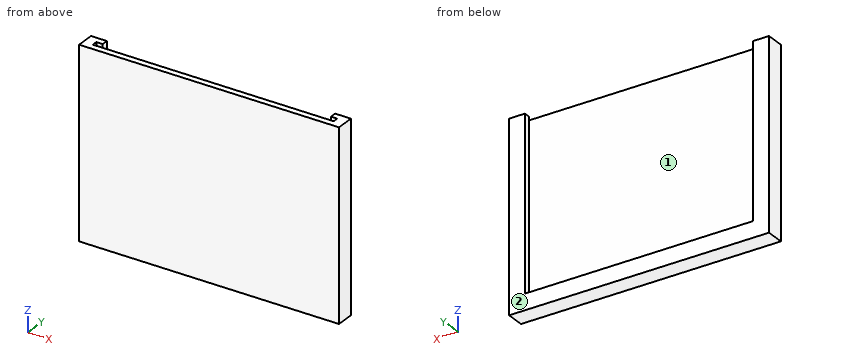
Autodesk Inventor part; units mm, degrees
ref_plane "YZ Plane" through (0, 0, 0) normal (1, 0, 0) x (0, 1, 0)
ref_plane "XZ Plane" through (0, 0, 0) normal (0, 1, 0) x (-1, 0, 0)
ref_plane "XY Plane" through (0, 0, 0) normal (0, 0, 1) x (1, 0, 0)
sketch "Szkic1" plane through (0, 0, 0) normal (0, 1, 0) x (-1, 0, 0)
  line L0 (7, 46.073) -> (-75, 46.073)
  line L1 (-75, 46.073) -> (-75, -13)
  line L2 (-75, -13) -> (7, -13)
  line L3 (7, -13) -> (7, 46.073)
  point P0 (0, 0)
  dimension "d0" = 82
  dimension "d1" = 59.073
extrude "Wyciągnięcie proste1" add sketch "Szkic1" along normal blind 2
sketch "Szkic2" plane through (0, 2, 0) normal (0, 1, 0) x (1, 0, 0)
  line L0 (75, -46.073) -> (75, 13)
  line L1 (75, 13) -> (-7, 13)
  line L2 (-7, 13) -> (-7, -46.073)
  line L3 (-7, -46.073) -> (75, -46.073)
  line L4 (-4, 10) -> (72, 10)
  line L5 (72, 10) -> (72, -43.073)
  line L6 (72, -43.073) -> (-4, -43.073)
  line L7 (-4, -43.073) -> (-4, 10)
  line L8 (-4, -43.073) -> (-4, -46.073)
  line L9 (72, -43.073) -> (72, -46.073)
  line L10 (-7, -46.073) -> (75, -46.073)
  point P0 (0, 0)
  dimension "d4" = 3
extrude "Wyciągnięcie proste2" add sketch "Szkic2" along normal blind 1.7 contours L3 L9 L5 L4 L7 L8 L2 L1 L0
sketch "Szkic3" plane through (0, 3.7, 0) normal (0, 1, 0) x (1, 0, 0)
  line L0 (75, 13) -> (-7, 13)
  line L1 (-7, 13) -> (-7, -46.073)
  line L2 (-7, -46.073) -> (-4, -46.073)
  line L3 (72, -46.073) -> (75, -46.073)
  line L4 (75, -46.073) -> (75, 13)
  line L5 (72, -46.073) -> (72, 10)
  line L6 (72, 10) -> (-4, 10)
  line L7 (-4, 10) -> (-4, -46.073)
  line L8 (-4, -46.073) -> (72, -46.073)
  line L9 (-2, 8) -> (70, 8)
  line L10 (70, 8) -> (70, -44.073)
  line L11 (70, -44.073) -> (-2, -44.073)
  line L12 (-2, -44.073) -> (-2, 8)
  line L13 (-2, -44.073) -> (-2, -46.073)
  line L14 (-7, -46.073) -> (75, -46.073)
  line L15 (70, -44.073) -> (70, -46.073)
  point P0 (0, 0)
  dimension "d7" = 2
extrude "Wyciągnięcie proste3" add sketch "Szkic3" along normal blind 2 contours L4 L3 L5 L6 L7 L2 L1 L0 | L8 L15 L10 L9 L12 L13 L7 L6 L5
properties part number "podstawka_na_pcb"
The model under review builds one solid part; all positions refer to its coordinate system, in mm. Face numbers are marked on the shaded views. Round coordinates to 2 decimals unless told otherwise and drop trailing zeros. Loops run counter-clockwise (first coordinate to the right, second up) from the corner with the lowest first, then second, coordinate; pieces in that order, holes last. Notation, with made-up numbers: (10, 12) - (68, 12) arc R21 cw to (68, 43) - close; hole circle Ø2 at (64, -39.5). An arc over 180 degrees is marked (long way). Use CSV: the item, a comma, the result in double quotes.
(1) Clearance check with flat-ended pins moving along their axes: P1, Ø10, axis at x = 1.5, z = -3, coming from the -Y side; P2, Ø2, axis at x = 65, z = -4, coming from the +Y side; P3, Ø1.6, axis at x = 33.5, y = 4.5, coming from the +Z side; P4, Ø0.5, axis at x = 34.5, y = 2.5, coming from the +Z side. State where each tip first meets the part, or that it passes through.
Working result:
P1,"stops at y = 0"
P2,"stops at y = 2"
P3,"stops at z = -8"
P4,"stops at z = -10"
(2) For line 1 (X direction, y = 3.9, z = 15.5); line 2 (X direction, y = 2.9, z = 10); line 3 (Y direction, x = 19, z = 23.5), list the stretches that pass through material, from the lowest coordinate up.
Working result:
line 1,"x = -7 to -2, 70 to 75"
line 2,"x = -7 to -4, 72 to 75"
line 3,"y = 0 to 2"
(3) Take a section at B-B, the plane y = 4.8. Give the boundary of the cut face in (x, z), plus the area to 3 significant figures.
Working result:
outline,"(-7, -13) - (75, -13) - (75, 46.07) - (70, 46.07) - (70, -8) - (-2, -8) - (-2, 46.07) - (-7, 46.07) - close"
area,"951 mm^2"
(4) The part is to be moulded in two halves that separate along X. For the marked faces 1 and 2, say which applies: pulls with the +X half, pulls with the -X half, needs draft (parallel to the pull), parting line crosses it, or undercut.
Working result:
face 1,"undercut"
face 2,"needs draft"
(5) Take a section at C-C, the plane x = 12.5. Give the boundary of the cut face in (y, z), plus the area to 3 significant figures.
Working result:
outline,"(0, -13) - (5.7, -13) - (5.7, -8) - (3.7, -8) - (3.7, -10) - (2, -10) - (2, 46.07) - (0, 46.07) - close"
area,"133 mm^2"
(6) Take a section at A-A, the plane z = 25.5. Give the boundary of the cut face in (x, y).
Working result:
outline,"(-7, 0) - (75, 0) - (75, 5.7) - (70, 5.7) - (70, 3.7) - (72, 3.7) - (72, 2) - (-4, 2) - (-4, 3.7) - (-2, 3.7) - (-2, 5.7) - (-7, 5.7) - close"
